Model file for the job. Use its own axes, mm. Face numbers are marked on the shaded views. A direction names the side the tool comes from. Coordinates: 2 decimals unless noted, no trailing zeros. Write each loop counter-clockwise with the first axis right and the second up, starting at its lowest first coordinate (ties: lowest second). Pieces come first, ordered by that corner, then holes. Notation, with made-up numbers: (36.5, 38) -> (56.5, 38) arc R16 ccw to (56.5, 69) -> close; hole circle Ø2 at (81.5, 13.5). An arc over 180 degrees is marked (long way). Answer as a JSON object with one key per item and string values. Group by question number.
from build123d import *

# Parameters (mm, degrees)
SKETCH1_R           = 1.5
BOSS_EXTRUDE1_DEPTH = 1.5
SKETCH2_R           = 3
SKETCH2_R_2         = 2.5
BOSS_EXTRUDE2_DEPTH = 2
SKETCH3_R           = 2.5
CUT_EXTRUDE1_DEPTH  = 0.5


with BuildPart() as part:
    # Sketch1 → Boss-Extrude1 (new body)
    with BuildSketch(Plane(origin=(0, 0, 0), x_dir=(1, 0, 0), z_dir=(0, 1, 0))):
        with BuildLine():
            Line((0.346153846, 2.97996267), (13.173076923, 1.489981335))
            ThreePointArc((13.173076923, 1.489981335), (14.5, 0), (13.173076923, -1.489981335))
            Line((13.173076923, -1.489981335), (0.346153846, -2.97996267))
            ThreePointArc((0.346153846, -2.97996267), (-3, 0), (0.346153846, 2.97996267))
        make_face()
        Circle(SKETCH1_R, mode=Mode.SUBTRACT)
    extrude(amount=BOSS_EXTRUDE1_DEPTH)

    # Sketch2 → Boss-Extrude2 (add)
    with BuildSketch(Plane(origin=(0, 1.5, 0), x_dir=(1, 0, 0), z_dir=(0, 1, 0))):
        Circle(SKETCH2_R)
        Circle(SKETCH2_R_2, mode=Mode.SUBTRACT)
    extrude(amount=BOSS_EXTRUDE2_DEPTH)

    # Sketch3 → Cut-Extrude1 (cut)
    with BuildSketch(Plane(origin=(0, 1.5, 0), x_dir=(1, 0, 0), z_dir=(0, 1, 0))):
        Circle(SKETCH3_R)
    extrude(amount=-CUT_EXTRUDE1_DEPTH, mode=Mode.SUBTRACT)


solid = part.part
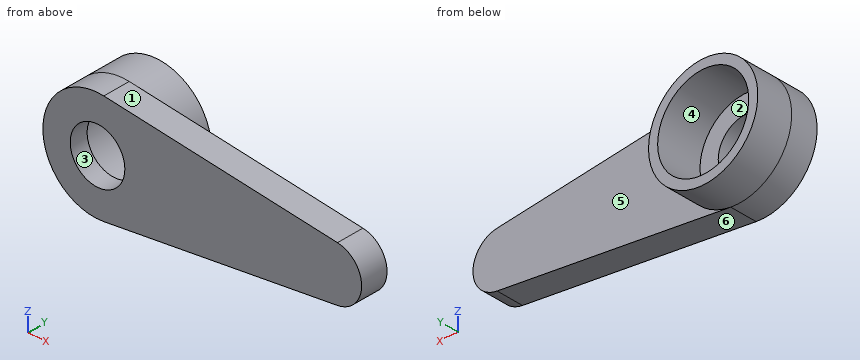
(1) Wall check: probe 1 along Z at (x, y) = (0, 0.75); probe 2 along Z at (x, y) = (0, 1.7). Give the ranges that are in metal, low to high.
(2) Cut at A-A on x = 0. List the corners of the cut face in (y, z), plus the area to 3 significant figures.
(3) Cut at C-C on y = 0.5. List the corners of the cut face in (x, z), plus the area to 3 significant figures.
(4) 3-axis set-ups, long thin cutter, end or side, ignore diameter. For the marked faces 1 and 2: which of +Z, -Z, +X, -X, +Y, -Y reach the whole face in a straight line?
(5) Cut at D-D on x = 8.5. List the corners of the cut face in (y, z), plus the area to 3 significant figures.
(6) Pull direction Z, two halves, no side cores. Call the marked faces 3, 4, 5 and 6: released by +Z, released by -Z, zero draft, split by the parting line, or undercut.
(7) Pin check, flat tip, straight feed: pin 1 (1.5 mm diameter, centred on y = 1.5, z = -1.5, fed in from +X). Stop position of the tip, or through.
(8) Cut at B-B on z = 0. List the corners of the cut face in (x, y), plus the area to 4 significant figures.
Results found:
{
 "1": {"probe 1": "z = -3 to -1.5, 1.5 to 3", "probe 2": "z = -3 to -2.5, 2.5 to 3"},
 "2": {"outline": "(0, -3) -> (3.5, -3) -> (3.5, -2.5) -> (1, -2.5) -> (1, -1.5) -> (0, -1.5) -> close; (0, 1.5) -> (1, 1.5) -> (1, 2.5) -> (3.5, 2.5) -> (3.5, 3) -> (0, 3) -> close", "area": "5.50 mm²"},
 "3": {"outline": "(0.35, -2.98) -> (13.17, -1.49) arc R1.5 ccw to (13.17, 1.49) -> (0.35, 2.98) arc R3 ccw (long way) to start; hole circle Ø3 at (0, 0)", "area": "69.5 mm²"},
 "4": {"face 1": "+Z, +X, +Y, -Y", "face 2": "+Y"},
 "5": {"outline": "(0, -2.03) -> (1.5, -2.03) -> (1.5, 2.03) -> (0, 2.03) -> close", "area": "6.10 mm²"},
 "6": {"face 3": "undercut", "face 4": "undercut", "face 5": "zero draft", "face 6": "released by -Z"},
 "7": {"pin 1": "stops at x = 14.3"},
 "8": {"outline": "(-3, 0) -> (-1.5, 0) -> (-1.5, 1) -> (-2.5, 1) -> (-2.5, 3.5) -> (-3, 3.5) -> close; (1.5, 0) -> (14.5, 0) -> (14.5, 1.5) -> (3, 1.5) -> (3, 3.5) -> (2.5, 3.5) -> (2.5, 1) -> (1.5, 1) -> close", "area": "22.75 mm²"}
}
